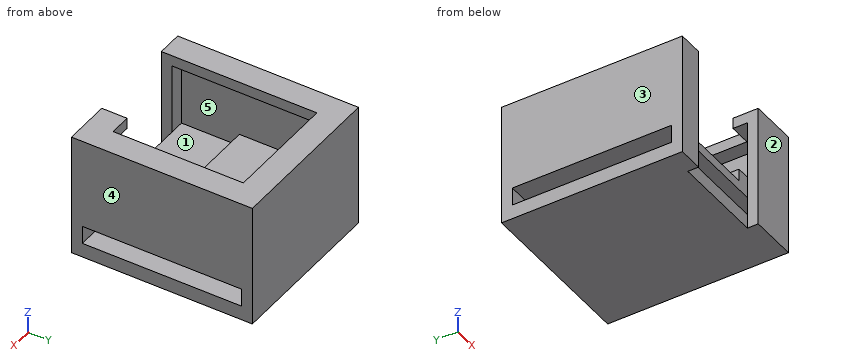
```python
from build123d import *

# Parameters (mm, degrees)
CROQUIS1_R               = 1.5
SALIENTE_EXTRUIR1_DEPTH  = 3
SALIENTE_EXTRUIR2_DEPTH  = 8
CROQUIS3_W               = 13
CROQUIS3_H               = 1.7
CORTAR_EXTRUIR1_DEPTH    = 8
CROQUIS5_W               = 3.5
CROQUIS5_H               = 11
CROQUIS5_W_2             = 6.5
SALIENTE_EXTRUIR3_DEPTH  = 1.5
SALIENTE_EXTRUIR4_DEPTH  = 1.5
CORTAR_EXTRUIR2_START    = -12.5
CORTAR_EXTRUIR2_DEPTH    = 3
SALIENTE_EXTRUIR10_DEPTH = 4.5
CORTAR_EXTRUIR3_START    = -22.8
CROQUIS12_W              = 2.5
CROQUIS12_H              = 22
CORTAR_EXTRUIR3_DEPTH    = 22.8


with BuildPart() as part:
    # Croquis1 → Saliente-Extruir1 (new body)
    with BuildSketch(Plane.XY):
        with BuildLine():
            Line((-55.603283504, 22.637490201), (-73.603283504, 19.937490201))
            ThreePointArc((-73.603283504, 19.937490201), (-74.822083019, 19.26473017), (-75.306602598, 17.959617496))
            Line((-75.306602598, 17.959617496), (-75.306602598, -5.318007663))
            Line((-75.306602598, -5.318007663), (-35.306602598, -5.318007663))
            Line((-35.306602598, -5.318007663), (-35.306602598, 17.959617496))
            ThreePointArc((-35.306602598, 17.959617496), (-35.791122177, 19.26473017), (-37.009921692, 19.937490201))
            Line((-37.009921692, 19.937490201), (-55.009921692, 22.637490201))
            ThreePointArc((-55.009921692, 22.637490201), (-55.306602598, 22.659617496), (-55.603283504, 22.637490201))
        make_face()
        with Locations((-71.306602598, 15.681992337)):
            Circle(CROQUIS1_R, mode=Mode.SUBTRACT)
        with Locations((-39.306602598, 15.681992337)):
            Circle(CROQUIS1_R, mode=Mode.SUBTRACT)
    extrude(amount=SALIENTE_EXTRUIR1_DEPTH)

    # Croquis2 → Saliente-Extruir2 (add)
    with BuildSketch(Plane.XY.offset(3)):
        Polygon((-66.706602598, -5.318007663), (-65.206602598, -5.318007663), (-65.206602598, 16.681992337), (-45.406602598, 16.681992337), (-45.406602598, -5.318007663), (-43.906602598, -5.318007663), (-43.906602598, 18.181992337), (-66.706602598, 18.181992337), align=None)
    extrude(amount=SALIENTE_EXTRUIR2_DEPTH)

    # Croquis3 → Cortar-Extruir1 (cut)
    with BuildSketch(Plane.XZ.offset(5.318007663)):
        with Locations((-58.706602598, 2.15)):
            Rectangle(CROQUIS3_W, CROQUIS3_H)
    extrude(amount=-CORTAR_EXTRUIR1_DEPTH, mode=Mode.SUBTRACT)

    # Croquis5 → Saliente-Extruir3 (add)
    with BuildSketch(Plane.XZ.offset(5.318007663)):
        with Locations((-64.956602598, 5.5)):
            Rectangle(CROQUIS5_W, CROQUIS5_H)
        with Locations((-47.156602598, 5.5)):
            Rectangle(CROQUIS5_W_2, CROQUIS5_H)
    extrude(amount=SALIENTE_EXTRUIR3_DEPTH)

    # Croquis6 → Saliente-Extruir4 (add)
    with BuildSketch(Plane.XY.offset(11)):
        Polygon((-63.206602598, -5.318007663), (-63.206602598, -6.818007663), (-66.706602598, -6.818007663), (-66.706602598, 18.181992337), (-43.906602598, 18.181992337), (-43.906602598, -6.818007663), (-50.406602598, -6.818007663), (-50.406602598, -3.318007663), (-47.406602598, -3.318007663), (-47.406602598, 14.681992337), (-63.206602598, 14.681992337), align=None)
    extrude(amount=SALIENTE_EXTRUIR4_DEPTH)

    # Croquis7 → Cortar-Extruir2 (cut)
    with BuildSketch(Plane.XY.offset(12.5).offset(CORTAR_EXTRUIR2_START)):
        Polygon((-66.706602598, -6.818007663), (-66.706602598, 18.181992337), (-43.906602598, 18.181992337), (-43.906602598, -6.818007663), (-20.536273409, -6.818007663), (-20.536273409, 28.419792756), (-79.716652243, 28.419792756), (-79.716652243, -6.818007663), align=None)
    extrude(amount=CORTAR_EXTRUIR2_DEPTH, mode=Mode.SUBTRACT)

    # Croquis11 → Saliente-Extruir10 (add)
    with BuildSketch(Plane(origin=(0, 0, 0), x_dir=(-1, 0, 0), z_dir=(0, 0, -1))):
        Polygon((66.706602598, 18.181992337), (43.906602598, 18.181992337), (43.906602598, -6.818007663), (50.406602598, -6.818007663), (50.406602598, -5.318007663), (63.206602598, -5.318007663), (63.206602598, -6.818007663), (66.706602598, -6.818007663), align=None)
    extrude(amount=SALIENTE_EXTRUIR10_DEPTH)

    # Croquis12 → Cortar-Extruir3 (cut)
    with BuildSketch(Plane(origin=(-43.906602598, 0, 0), x_dir=(0, 0, -1), z_dir=(1, 0, 0)).offset(CORTAR_EXTRUIR3_START)):
        with Locations((1.25, 5.681992337)):
            Rectangle(CROQUIS12_W, CROQUIS12_H)
    extrude(amount=CORTAR_EXTRUIR3_DEPTH, mode=Mode.SUBTRACT)


solid = part.part
```
Part model, mm, in its own coordinate system. Face numbers are marked on the shaded views. A direction names the side the tool comes from. Round coordinates to 2 decimals unless told otherwise and drop trailing zeros. Order: outer loops, then holes, each group sorted by start corner. A loop starts at its lowest first (then second) coordinate and runs counter-clockwise, first axis right, second up. Notation, with made-up numbers: M 6.25,78.25 L 18.25,78.25 A28 ccw 18.25,99.25 Z; hole C 68.5,-25 d11. An arc over 180 degrees is marked long. Answer in a Markdown table with one row per item. Add a question column.
Q1. Cut at A-A on y = 1.5. Give the cut face in (x, z).
Q2. 3-axis set-ups, long thin cutter, end or side, ignore diameter. For the marked faces 4 and 5: which of +Z, -Z, +X, -X, +Y, -Y reach the whole face in a straight line?
Q3. Cut at C-C on x = -57.25. Give the cut face in (y, z).
Q4. Cut at D-D on z = 10. Give the cut face in (x, y).
Q5. Cut at B-B on z = -1.75. Give the cut face in (x, y), and give its area (3 significant figures).
Q6. Wall check: L1, parallel to Z at x = -53.75, y = 16; L2, parallel to X at y = -3.5, z = 9.5; L3, parallel to Z at x = -49.25, y = 9.75. Give the ranges that are in metal, low to high. Write a range as from..to.
Q7. Pin check, flat tips, straight feed: pin 1 (3 mm diameter, centred on x = -56.5, z = 2.5, fed in from -Y); pin 2 (3 mm diameter, centred on x = -52.5, y = 7, fed in from +Z); pin 3 (0.8 mm diameter, centred on x = -53.5, z = -1, fed in from -Y). Stop position of each tip, or through.
Q8. Mould opens along X. For the marked faces 1, 2 and 3 say: +X half, -X half, draft (parallel to the pull), parting line (faces both ways), or undercut.
Established:
| question | item | result |
|---|---|---|
| 1 | outline | M -66.71,-4.5 L -43.91,-4.5 L -43.91,-2.5 L -66.71,-2.5 Z; M -66.71,0 L -43.91,0 L -43.91,12.5 L -47.41,12.5 L -47.41,11 L -45.41,11 L -45.41,3 L -52.21,3 L -52.21,1.3 L -65.21,1.3 L -65.21,11 L -63.21,11 L -63.21,12.5 L -66.71,12.5 Z |
| 2 | face 4 | +Z, -Z, +X, +Y, -Y |
| 2 | face 5 | none |
| 3 | outline | M -5.32,-4.5 L 18.18,-4.5 L 18.18,12.5 L 14.68,12.5 L 14.68,11 L 16.68,11 L 16.68,3 L 2.68,3 L 2.68,1.3 L -5.32,1.3 L -5.32,0 L 16.68,0 L 16.68,-2.5 L -5.32,-2.5 Z |
| 4 | outline | M -66.71,-6.82 L -63.21,-6.82 L -63.21,-5.32 L -65.21,-5.32 L -65.21,16.68 L -45.41,16.68 L -45.41,-5.32 L -50.41,-5.32 L -50.41,-6.82 L -43.91,-6.82 L -43.91,18.18 L -66.71,18.18 Z |
| 5 | outline | M -66.71,-6.82 L -63.21,-6.82 L -63.21,-5.32 L -66.71,-5.32 Z; M -66.71,16.68 L -43.91,16.68 L -43.91,18.18 L -66.71,18.18 Z; M -50.41,-6.82 L -43.91,-6.82 L -43.91,-5.32 L -50.41,-5.32 Z |
| 5 | area | 49.2 mm2 |
| 6 | L1 | z = -4.5..-2.5, 0..3, 11..12.5 |
| 6 | L2 | x = -66.71..-65.21, -45.41..-43.91 |
| 6 | L3 | z = -4.5..-2.5, 0..3 |
| 7 | pin 1 | stops at y = -5.32 |
| 7 | pin 2 | stops at z = 3 |
| 7 | pin 3 | stops at y = 16.68 |
| 8 | face 1 | undercut |
| 8 | face 2 | draft |
| 8 | face 3 | -X half |
